Could you check a few things on this model? Use its own coordinates, in mm. Face numbers are marked on the shaded views. A direction names the side the tool comes from. Coordinates: 2 decimals unless noted, no trailing zeros. Write each loop counter-clockwise with the first axis right and the second up, starting at its lowest first coordinate (ties: lowest second). Pieces come first, ordered by that corner, then holes. Notation, with made-up numbers: (-34.5, 81.5) - (-14.5, 81.5) arc R12 cw to (-14.5, 102.5) - close; hole circle Ø4 at (1, 54). An arc over 180 degrees is marked (long way). Answer as a JSON object with one key per item and string values. Group by question number.
1) If we section it at C-C (z = 2): Write out the boundary of the cut face in (x, y).
2) If we section it at A-A (x = 0): Write out the boundary of the cut face in (y, z) (3 decimals), plus the area to 3 significant figures.
3) We'd pull the mould along Y, two halves only. Please class the marked faces 6, 7, 8 and 9: released by +Y, released by -Y, zero draft, split by the parting line, or undercut.
4) If we section it at B-B (y = 0): Write out the boundary of the cut face in (x, z) (3 decimals).
5) Will these pins go through, and if not, where does the flat tip stop? pin 1 Ø8 at (x, y) = (-5.5, 6) entering from -Z; pin 2 Ø6 at (y, z) = (1, 4.5) entering from +X; pin 3 Ø1 at (y, z) = (4.5, -5.5) entering from +X; pin 4 Ø3.5 at (x, y) = (0, 0) entering from -Z.
6) On a 3-axis mill with a long thin cutter (end or side, diameter ignored), from which of +Z, -Z, +X, -X, +Y, -Y can I reach the whole of each face in a straight line? I mean the marked faces 1, 2, 3, 4 and 5. Say none if no direction works.
7) Please list where these lines run through material, in increasing order: line 1 along X through (y, z) = (0, 8.75); line 2 along Y through (x, z) = (0, 7.75); line 3 along Z through (x, y) = (6.75, 1.25) (3 decimals).
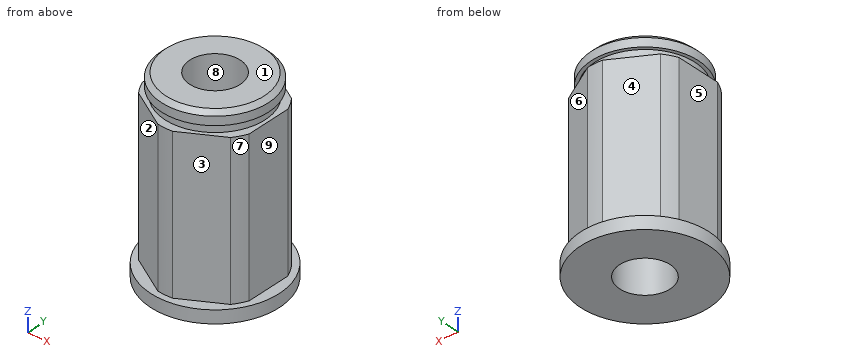
```python
from build123d import *

# Parameters (mm, degrees)
SKETCH1_R               = 6.35
BASIC_ROD_DEPTH         = 9.779
BASIC_ROD_DEPTH_BACK    = 9.779
THEX_DEPTH              = 9.779
SKETCH2_R               = 2.9972
INTERNAL_CUT_DEPTH      = 13.319
INTERNAL_CUT_DEPTH_BACK = 10.779
SKETCH9_R               = 7.62
SKETCH9_R_2             = 2.9972
BOSS_EXTRUDE1_DEPTH     = 1.524


with BuildPart() as part:
    # Sketch1 → Basic Rod (new body, two sides)
    with BuildSketch(Plane.XY) as basic_rod_sk:
        Circle(SKETCH1_R)
    extrude(amount=BASIC_ROD_DEPTH)
    extrude(basic_rod_sk.sketch, amount=-BASIC_ROD_DEPTH_BACK)

    # Sketch8 → THex (add, symmetric)
    with BuildSketch(Plane.XY):
        with BuildLine():
            Line((-0.888411378, 6.819423871), (-5.461588622, 4.179098758))
            ThreePointArc((-5.461588622, 4.179098758), (-5.955700003, 3.438525), (-6.35, 2.640325113))
            Line((-6.35, 2.640325113), (-6.35, -2.640325113))
            ThreePointArc((-6.35, -2.640325113), (-5.955700003, -3.438525), (-5.461588622, -4.179098758))
            Line((-5.461588622, -4.179098758), (-0.888411378, -6.819423871))
            ThreePointArc((-0.888411378, -6.819423871), (0, -6.87705), (0.888411378, -6.819423871))
            Line((0.888411378, -6.819423871), (5.461588622, -4.179098758))
            ThreePointArc((5.461588622, -4.179098758), (5.955700003, -3.438525), (6.35, -2.640325113))
            Line((6.35, -2.640325113), (6.35, 2.640325113))
            ThreePointArc((6.35, 2.640325113), (5.955700003, 3.438525), (5.461588622, 4.179098758))
            Line((5.461588622, 4.179098758), (0.888411378, 6.819423871))
            ThreePointArc((0.888411378, 6.819423871), (0, 6.87705), (-0.888411378, 6.819423871))
        make_face()
    extrude(amount=THEX_DEPTH, both=True)

    # Sketch7 → 1stSnapRing (revolve)
    with BuildSketch(Plane(origin=(0, 0, 0), x_dir=(0, 0, -1), z_dir=(1, 0, 0))):
        Polygon((-9.779, 5.9436), (-10.795, 5.9436), (-10.795, 6.35), (-11.811, 6.35), (-12.319, 5.842), (-12.319, 0), (-9.779, 0), align=None)
    revolve(axis=Axis((0, 0, -38.2778), (0, 0, 1)))

    # Sketch2 → Internal Cut (cut, two sides)
    with BuildSketch(Plane.XY) as internal_cut_sk:
        Circle(SKETCH2_R)
    extrude(amount=INTERNAL_CUT_DEPTH, mode=Mode.SUBTRACT)
    extrude(internal_cut_sk.sketch, amount=-INTERNAL_CUT_DEPTH_BACK, mode=Mode.SUBTRACT)

    # Sketch9 → Boss-Extrude1 (add)
    with BuildSketch(Plane(origin=(0, 0, -9.779), x_dir=(-1, 0, 0), z_dir=(0, 0, -1))):
        Circle(SKETCH9_R)
        Circle(SKETCH9_R_2, mode=Mode.SUBTRACT)
    extrude(amount=-BOSS_EXTRUDE1_DEPTH)


solid = part.part
```
Here are the results:
{
 "1": {"outline": "(-6.35, -2.64) arc R6.88 ccw to (-5.46, -4.18) - (-0.89, -6.82) arc R6.88 ccw to (0.89, -6.82) - (5.46, -4.18) arc R6.88 ccw to (6.35, -2.64) - (6.35, 2.64) arc R6.88 ccw to (5.46, 4.18) - (0.89, 6.82) arc R6.88 ccw to (-0.89, 6.82) - (-5.46, 4.18) arc R6.88 ccw to (-6.35, 2.64) - close; hole circle Ø5.99 at (0, 0)"},
 "2": {"outline": "(-7.62, -9.779) - (-2.997, -9.779) - (-2.997, 12.319) - (-5.842, 12.319) - (-6.35, 11.811) - (-6.35, 10.795) - (-5.944, 10.795) - (-5.944, 9.779) - (-6.877, 9.779) - (-6.877, -8.255) - (-7.62, -8.255) - close; (2.997, -9.779) - (7.62, -9.779) - (7.62, -8.255) - (6.877, -8.255) - (6.877, 9.779) - (5.944, 9.779) - (5.944, 10.795) - (6.35, 10.795) - (6.35, 11.811) - (5.842, 12.319) - (2.997, 12.319) - close", "area": "170 mm²"},
 "3": {"face 6": "released by +Y", "face 7": "released by -Y", "face 8": "undercut", "face 9": "zero draft"},
 "4": {"outline": "(-7.62, -9.779) - (-2.997, -9.779) - (-2.997, 12.319) - (-5.842, 12.319) - (-6.35, 11.811) - (-6.35, 10.795) - (-5.944, 10.795) - (-5.944, 9.779) - (-6.35, 9.779) - (-6.35, -8.255) - (-7.62, -8.255) - close; (2.997, -9.779) - (7.62, -9.779) - (7.62, -8.255) - (6.35, -8.255) - (6.35, 9.779) - (5.944, 9.779) - (5.944, 10.795) - (6.35, 10.795) - (6.35, 11.811) - (5.842, 12.319) - (2.997, 12.319) - close"},
 "5": {"pin 1": "stops at z = -9.78", "pin 2": "stops at x = 6.35", "pin 3": "stops at x = 5.59", "pin 4": "passes through"},
 "6": {"face 1": "+Z, +X, -X, +Y, -Y", "face 2": "+Z, -X, -Y", "face 3": "+Z, +X, -Y", "face 4": "+Z, -X, +Y", "face 5": "+Z, -X, +Y, -Y"},
 "7": {"line 1": "x = -6.35 to -3, 3 to 6.35", "line 2": "y = -6.88 to -3, 3 to 6.88", "line 3": "z = -9.779 to -8.255"}
}
